```python
from build123d import *

# Parameters (mm, degrees)
SKETCH1_R           = 40
SKETCH1_R_2         = 5
BOSS_EXTRUDE3_DEPTH = 10
SKETCH3_R           = 25
SKETCH3_R_2         = 22
BOSS_EXTRUDE4_DEPTH = 50.8
SKETCH9_R           = 10
CUT_EXTRUDE1_DEPTH  = 100


with BuildPart() as part:
    # Sketch1 → Boss-Extrude3 (new body)
    with BuildSketch(Plane.XY):
        Circle(SKETCH1_R)
        with Locations((0, -32)):
            Circle(SKETCH1_R_2, mode=Mode.SUBTRACT)
        with Locations(Location((0, 32, 0), (0, 0, 180))):
            Circle(SKETCH1_R_2, mode=Mode.SUBTRACT)
        with Locations((-32, 0)):
            Circle(SKETCH1_R_2, mode=Mode.SUBTRACT)
        with Locations(Location((32, 0, 0), (0, 0, 180))):
            Circle(SKETCH1_R_2, mode=Mode.SUBTRACT)
    extrude(amount=BOSS_EXTRUDE3_DEPTH)

    # Sketch3 → Boss-Extrude4 (add)
    with BuildSketch(Plane.XY.offset(10)):
        Circle(SKETCH3_R)
        Circle(SKETCH3_R_2, mode=Mode.SUBTRACT)
    extrude(amount=BOSS_EXTRUDE4_DEPTH)

    # Sketch9 → Cut-Extrude1 (cut)
    with BuildSketch(Plane(origin=(0, 0, 0), x_dir=(-1, 0, 0), z_dir=(0, 0, -1))):
        Circle(SKETCH9_R)
    extrude(amount=-CUT_EXTRUDE1_DEPTH, mode=Mode.SUBTRACT)


solid = part.part
```
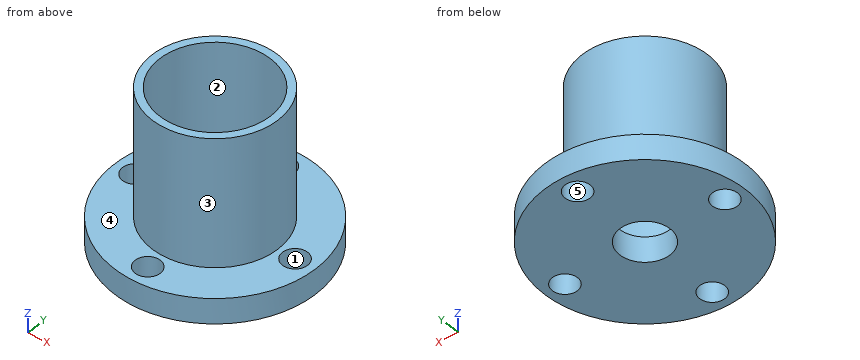
Verification items for the finished model (mm, model axes). Face numbers are marked on the shaded views. A direction names the side the tool comes from. Round coordinates to 2 decimals unless told otherwise and drop trailing zeros. Write each loop counter-clockwise with the first axis right and the second up, starting at its lowest first coordinate (ties: lowest second). Pieces come first, ordered by that corner, then holes. Notation, with made-up numbers: (72.5, 84.25) - (81.5, 84.25) arc R27 ccw to (81.5, 115.25) - close; hole circle Ø5 at (52.5, 2). An arc over 180 degrees is marked (long way). Answer as a JSON object with one key per item and string values. Group by question number.
Q1. Section check B-B, the plane x = 32. Enter the section's corners in (y, z).
Q2. Go/stop test with flat-tipped pins: pin 1 Ø9 at (x, y) = (0, -32) entering from +Z; pin 2 Ø5 at (x, y) = (-7.5, 12.5) entering from +Z; pin 3 Ø12 at (y, z) = (-1.5, 50.5) entering from +X; pin 4 Ø1 at (y, z) = (15.5, 11.5) entering from +X. Record where each tip stops, or that it passes through.
Q3. Section check A-A, the plane y = 0. Enter the section's corners in (x, z).
Q4. Tool access check on the marked faces 1 and 2. Record the directions out of +Z, -Z, +X, -X, +Y, -Y that give a thin tool (end or side, any length) a straight path to the whole face; none if there is none.
Q5. Section check D-D, the plane z = 7. Enter the section's corners in (x, y), plus the area to 3 significant figures.
Q6. Thickness scan on line 1 (Y direction, x = 0, z = 6.25); line 2 (Z direction, x = 25, y = -15); line 3 (X direction, y = 10, z = 58.5). Record the ranges inside material, lowest first.
Q7. Mould release check, pull along Y, two halves, no side actions. Record for the marked faces 3, 4 and 5: released by +Y, released by -Y, zero draft, split by the parting line, or undercut.
Found:
{
 "1": {"outline": "(-24, 0) - (-5, 0) - (-5, 10) - (-24, 10) - close; (5, 0) - (24, 0) - (24, 10) - (5, 10) - close"},
 "2": {"pin 1": "passes through", "pin 2": "stops at z = 10", "pin 3": "stops at x = 25", "pin 4": "stops at x = 20"},
 "3": {"outline": "(-40, 0) - (-37, 0) - (-37, 10) - (-40, 10) - close; (-27, 0) - (-10, 0) - (-10, 10) - (-22, 10) - (-22, 60.8) - (-25, 60.8) - (-25, 10) - (-27, 10) - close; (10, 0) - (27, 0) - (27, 10) - (25, 10) - (25, 60.8) - (22, 60.8) - (22, 10) - (10, 10) - close; (37, 0) - (40, 0) - (40, 10) - (37, 10) - close"},
 "4": {"face 1": "+Z, -Z", "face 2": "+Z"},
 "5": {"outline": "circle Ø80 at (0, 0); hole circle Ø10 at (-32, 0); hole circle Ø20 at (0, 0); hole circle Ø10 at (0, -32); hole circle Ø10 at (0, 32); hole circle Ø10 at (32, 0)", "area": "4,400 mm^2"},
 "6": {"line 1": "y = -40 to -37, -27 to -10, 10 to 27, 37 to 40", "line 2": "z = 0 to 10", "line 3": "x = -22.91 to -19.6, 19.6 to 22.91"},
 "7": {"face 3": "split by the parting line", "face 4": "zero draft", "face 5": "undercut"}
}
